Design review of the part shown in the three views and the two pictorial views. Dimensions are in mm from the part's minimum x, y and z. Round coordinates to 2 decimals unless told otherwise and drop trailing zeros. Loops run counter-clockwise (first coordinate to the right, second up) from the corner with the lowest first, then second, coordinate; pieces in that order, holes last. Notation, with made-up numbers: (5.25, 66.25) -> (30.25, 66.25) arc R20 ccw to (30.25, 99.25) -> close; hole circle Ø1 at (-35, 46.25). An arc over 180 degrees is marked (long way). Use a Markdown table: item, result. Add a question column.
1) Mouldability with a two-part tool opening along Y and no side actions: class the marked faces 1, 2 and 3 as released by +Y, released by -Y, zero draft, split by the parting line, or undercut.
2) Consider section C-C on z = 59. Give the boundary of the cut face in (x, y).
3) Consider section B-B on z = 32.5. Give the boundary of the cut face in (x, y), plus the area to 3 significant figures.
4) Insertion check: pin 1 (3 mm diameter, centred on y = 151.5, z = 33.5, fed in from +X); pin 2 (6 mm diameter, centred on y = 93, z = 29, fed in from +X). Each pin has a flat end and moves straight along its axis. Give the tip position at first contact, or say it passes through.
5) Consider section A-A on x = 13. Give the boundary of the cut face in (y, z), plus the area to 3 significant figures.
6) Wall thickness on probe 1 along Y at (x, z) = (48.5, 54); probe 2 along Z at (x, y) = (33.5, 49); probe 3 along X at (y, z) = (9, 45): over which ranges is each line inside the solid? List them lowest first.
7) Consider section D-D on y = 42. Give the boundary of the cut face in (x, z).
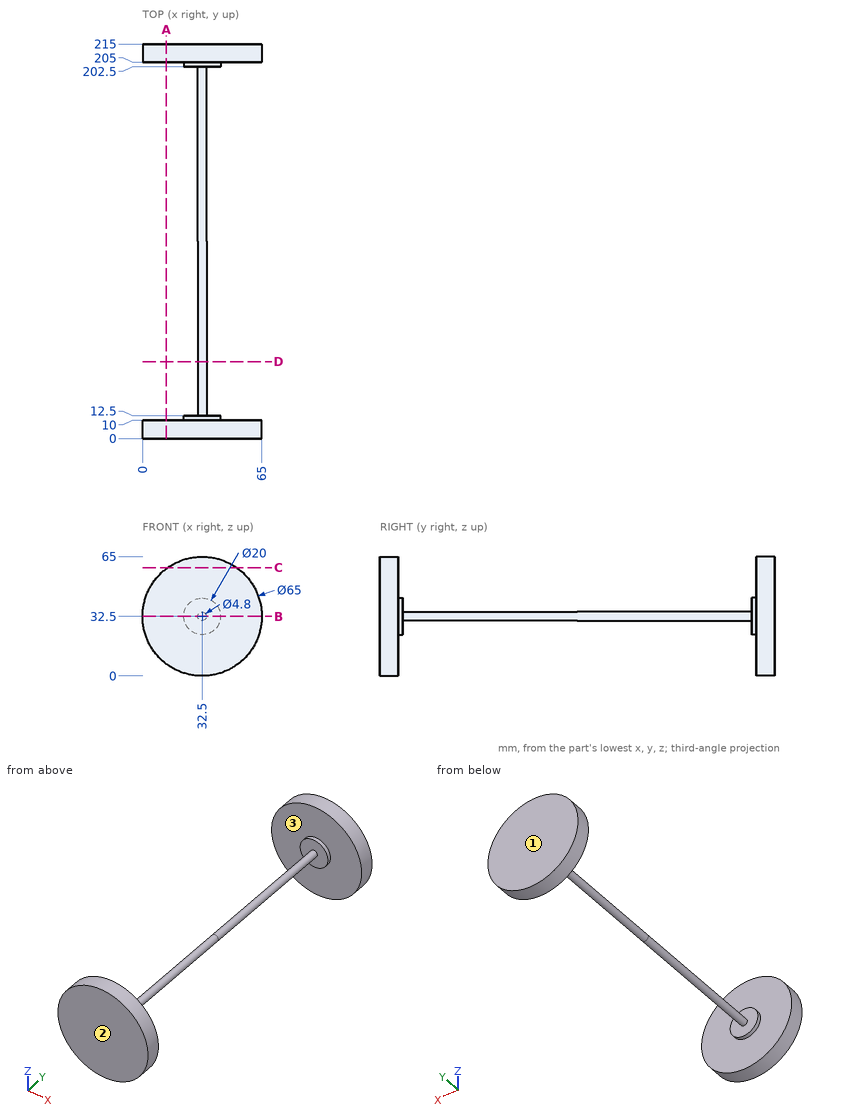
Result set:
| question | item | result |
|---|---|---|
| 1 | face 1 | released by +Y |
| 1 | face 2 | released by -Y |
| 1 | face 3 | undercut |
| 2 | outline | (13.69, 0) -> (51.31, 0) -> (51.31, 10) -> (13.69, 10) -> close; (13.69, 205) -> (51.31, 205) -> (51.31, 215) -> (13.69, 215) -> close |
| 3 | outline | (0, 0) -> (65, 0) -> (65, 10) -> (42.5, 10) -> (42.5, 12.5) -> (34.9, 12.5) -> (34.9, 202.5) -> (42.5, 202.5) -> (42.5, 205) -> (65, 205) -> (65, 215) -> (0, 215) -> (0, 205) -> (22.5, 205) -> (22.5, 202.5) -> (30.1, 202.5) -> (30.1, 12.5) -> (22.5, 12.5) -> (22.5, 10) -> (0, 10) -> close |
| 3 | area | 2,310 mm2 |
| 4 | pin 1 | x = 34.9 |
| 4 | pin 2 | x = 34.85 |
| 5 | outline | (0, 6.5) -> (10, 6.5) -> (10, 58.5) -> (0, 58.5) -> close; (205, 6.5) -> (215, 6.5) -> (215, 58.5) -> (205, 58.5) -> close |
| 5 | area | 1,040 mm2 |
| 6 | probe 1 | 0 to 10, 205 to 215 |
| 6 | probe 2 | 30.32 to 34.68 |
| 6 | probe 3 | 2.5 to 62.5 |
| 7 | outline | circle Ø4.8 at (32.5, 32.5) |
